Could you check a few things on this model? Use its own coordinates, in mm. A direction names the side the tool comes from. Give positions to 0.01 mm unless a question says otherwise; leave off trailing zeros. Order: outer loops, then holes, each group sorted by start corner. A loop starts at its lowest first (then second) coordinate and runs counter-clockwise, first axis right, second up.
(1) If I drill on probe 1 along Z at (x, y) = (522, -432.5); probe 2 along X at (y, z) = (-318.5, 235), over which ranges is the centre line in solid material (lowest first)?
(2) Imagine slicing it at C-C, the plane y = -64. Write out the boundary of the cut face in (x, z), then the cut area to 3 significant figures.
(3) Imagine slicing it at B-B, the plane z = 637. Write out the boundary of the cut face in (x, y).
(4) Will these pins go through, and if not, where does the flat tip stop? pin 1 (9 mm diameter, centred on y = 16.5, z = 429.5, fed in from -X); pin 2 (9 mm diameter, centred on y = 13, z = 342.5, fed in from +X).
(5) Imagine slicing it at A-A, the plane x = 88.5. Write out the boundary of the cut face in (y, z), then the cut area to 3 significant figures.
(6) Imagine slicing it at D-D, the plane x = 399. Write out the boundary of the cut face in (y, z).
(7) On a 3-axis mill with a long thin cutter (end or side, diameter ignored), from which of +Z, -Z, +X, -X, +Y, -Y can I reach the whole of each face in a straight line? I mean faces 1 (the flat face through (463.69, -320.65, 367.66)), 2 (the flat face through (15, 15, 368)), 3 (the flat face through (445.72, -318.1, 364.69)). Say none if no direction works.
(8) If we mould it in two halves opening along X, with no side actions, what happens to faces 4 (the flat face through (-450.632, -293.636, 367.662)), 5 (the flat face through (512, -435, 696)), 6 (the flat face through (470.7, -300.68, 364.69))? For each: released by +X, released by -X, zero draft, split by the parting line, or undercut.
from build123d import *

# Parameters (mm, degrees)
F1_DEPTH = 30
F3_DEPTH = 333
F5_DEPTH = 333


with BuildPart() as f1:
    # F0 (on Top) → F1 (new body)
    with BuildSketch(Plane.XY):
        Polygon((-297.3889, 0), (0, 0), (297.3889, 0), (556.8289580754, -556.371), (584.0181916865, -543.6924521478), (316.5010078242, 30), (0, 30), (-316.5010078242, 30), (-584.0181916865, -543.6924521478), (-556.8289580754, -556.371), align=None)
    extrude(amount=F1_DEPTH)

    # F2 (on face) → F3 (join)
    with BuildSketch(Plane.XY.offset(30)):
        Polygon((-15, 0), (0, 0), (15, 0), (15, 30), (-15, 30), align=None)
    extrude(amount=F3_DEPTH)

    # F4 (on face) → F5 (join)
    with BuildSketch(Plane.XY.offset(30)):
        Polygon((-437.2281658224, -299.886273315), (-464.4173994335, -287.2077254628), (-477.0959472857, -314.3969590739), (-449.9067136746, -327.0755069261), align=None)
    extrude(amount=F5_DEPTH)

    # F6: F1 across plane


with BuildPart() as f1_1:
    add(f1.part)
    add(f1.part.mirror(Plane.YZ))

    # F7: F1 across face


with BuildPart() as f1_2:
    add(f1_1.part)
    add(f1_1.part.mirror(Plane(origin=(0, 15, 363), x_dir=(1, 0, 0), z_dir=(0, 0, 1))))


solid = f1_2.part
Answer block:
1. probe 1: z = 0 to 30, 696 to 726
1. probe 2: x = -468.3 to -445.91, 445.91 to 468.3
2. outline: (-360.33, 0) - (-327.23, 0) - (-327.23, 30) - (-360.33, 30) - close; (-360.33, 696) - (-327.23, 696) - (-327.23, 726) - (-360.33, 726) - close; (327.23, 0) - (360.33, 0) - (360.33, 30) - (327.23, 30) - close; (327.23, 696) - (360.33, 696) - (360.33, 726) - (327.23, 726) - close
2. area: 3,970 mm2
3. outline: (-477.1, -314.4) - (-449.91, -327.08) - (-437.23, -299.89) - (-464.42, -287.21) - close; (-15, 0) - (15, 0) - (15, 30) - (-15, 30) - close; (437.23, -299.89) - (449.91, -327.08) - (477.1, -314.4) - (464.42, -287.21) - close
4. pin 1: stops at x = -15
4. pin 2: stops at x = 15
5. outline: (0, 0) - (30, 0) - (30, 30) - (0, 30) - close; (0, 696) - (30, 696) - (30, 726) - (0, 726) - close
5. area: 1,800 mm2
6. outline: (-217.91, 0) - (-146.92, 0) - (-146.92, 30) - (-217.91, 30) - close; (-217.91, 696) - (-146.92, 696) - (-146.92, 726) - (-217.91, 726) - close
7. face 1: +X, -Y
7. face 2: +X, +Y, -Y
7. face 3: +Z, -Z, -Y
8. face 4: undercut
8. face 5: zero draft
8. face 6: released by +X
